```python
from build123d import *

# Parameters (mm, degrees)
EXTRUDE_1_DEPTH      = 1.4
EXTRUDE_1_DEPTH_BACK = 1.935048816
MM_1_D               = 1
MM_1_DEPTH           = 3.69956969
MM_1_TIP             = 0.30043031
MM_2_D               = 1
MM_2_DEPTH           = 3.69956969
MM_2_TIP             = 0.30043031
EXTRUDE_4_DEPTH      = 4
EXTRUDE_4_DEPTH_BACK = 7
CUT_EXTRUDE_4_DEPTH  = 4


with BuildPart() as part:
    # 草图1 → 凸台-拉伸1 (new body, two sides)
    with BuildSketch(Plane.XY) as extrude_1_sk:
        with BuildLine():
            Line((-14, 10.976009084), (64.784112274, 10.976009084))
            ThreePointArc((64.784112274, 10.976009084), (69.784112274, 5.976009084), (64.784112274, 0.976009084))
            Line((64.784112274, 0.976009084), (-14, 0.976009084))
            ThreePointArc((-14, 0.976009084), (-19, 5.976009084), (-14, 10.976009084))
        make_face()
        with BuildLine():
            Line((21.676320512, 3.476009084), (-1.323679488, 3.476009084))
            ThreePointArc((-1.323679488, 3.476009084), (-3.823679488, 5.976009084), (-1.323679488, 8.476009084))
            Line((-1.323679488, 8.476009084), (21.676320512, 8.476009084))
            ThreePointArc((21.676320512, 8.476009084), (24.176320512, 5.976009084), (21.676320512, 3.476009084))
        make_face(mode=Mode.SUBTRACT)
    extrude(amount=EXTRUDE_1_DEPTH)
    extrude(extrude_1_sk.sketch, amount=-EXTRUDE_1_DEPTH_BACK)

    # 大小mm 暗销孔1
    with Locations(Plane(origin=(0, 0, -1.935048816), x_dir=(-1, 0, 0), z_dir=(0, 0, -1))):
        with Locations((14, 5.976009084)):
            Hole(MM_1_D / 2, depth=MM_1_DEPTH)
            with Locations((0, 0, -(MM_1_DEPTH + MM_1_TIP / 2))):  # 118° drill point
                Cone(0, MM_1_D / 2, MM_1_TIP, mode=Mode.SUBTRACT)

    # 大小mm 暗销孔2
    with Locations(Plane(origin=(0, 0, -1.935048816), x_dir=(-1, 0, 0), z_dir=(0, 0, -1))):
        with Locations((-64.784112274, 5.976009084)):
            Hole(MM_2_D / 2, depth=MM_2_DEPTH)
            with Locations((0, 0, -(MM_2_DEPTH + MM_2_TIP / 2))):  # 118° drill point
                Cone(0, MM_2_D / 2, MM_2_TIP, mode=Mode.SUBTRACT)

    # 草图11 → 凸台-拉伸4 (add, two sides)
    with BuildSketch(Plane.XY.offset(1.4)) as extrude_4_sk:
        with BuildLine():
            Line((64.784112274, 10.976009084), (75.11027427, 10.181945777))
            Line((75.11027427, 10.181945777), (68.706480161, 6.265649051))
            Line((68.706480161, 6.265649051), (69.231074418, 4.88985116))
            Line((69.231074418, 4.88985116), (75.876804715, 9.001268784))
            Line((75.876804715, 9.001268784), (76.348764637, 8.189866665))
            Line((76.348764637, 8.189866665), (64.784112274, 0.976009084))
            ThreePointArc((64.784112274, 0.976009084), (65.998123298, 5.976009084), (64.784112274, 10.976009084))
        make_face()
    extrude(amount=EXTRUDE_4_DEPTH)
    extrude(extrude_4_sk.sketch, amount=-EXTRUDE_4_DEPTH_BACK)

    # 草图12 → 切除-拉伸4 (cut)
    with BuildSketch(Plane.XY.offset(1.4)):
        Polygon((69.702654004, 6.874867944), (68.706480161, 6.265649051), (69.231074418, 4.88985116), (69.722566431, 5.193915399), (71.19681176, 6.105965386), align=None)
        Polygon((64.784112274, 0.976009084), (69.274656978, 3.777143865), (71.000307029, 3.200660754), (64.195477274, -1.252602435), align=None)
    extrude(amount=-CUT_EXTRUDE_4_DEPTH, mode=Mode.SUBTRACT)


solid = part.part
```
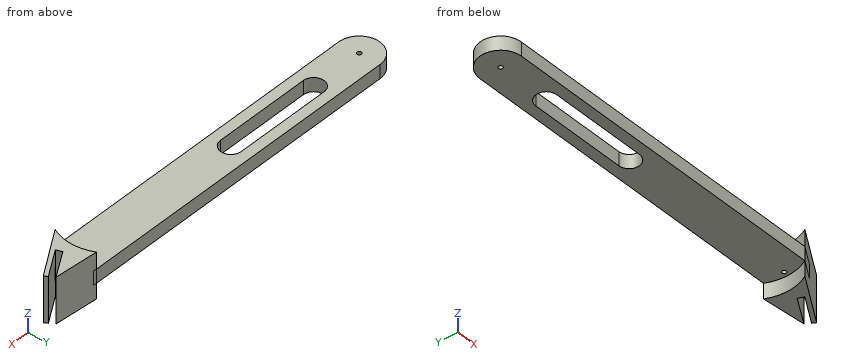
Verification items for the finished model (mm, model axes). Round coordinates to 2 decimals unless told otherwise and drop trailing zeros. Write each loop counter-clockwise with the first axis right and the second up, starting at its lowest first coordinate (ties: lowest second). Pieces come first, ordered by that corner, then holes.
1. Section check A-A on x = 9.5. Enter the section's corners in (y, z).
2. Gauge pin test, flat ends, axial feed: P1, Ø2, axis at x = 55, y = 4, coming from the -Z side; P2, Ø3, axis at y = 7.5, z = 3.5, coming from the +X side; P3, Ø3, axis at y = 2.5, z = 3, coming from the -X side; P4, Ø3, axis at y = 3.5, z = 0, coming from the -X side. Record the tip position at first contact, or that the pin passes through.
3. Scan lines: L1, parallel to Y at x = -14, z = 0.6; L2, parallel to Z at x = 17.5, y = 8.75; L3, parallel to X at y = 5.75, z = -4.25. Record each from-to range of solid material in increasing order.
4. Section check B-B on z = 2.75. Enter the section's corners in (x, y).
Answer:
1. outline: (0.98, -1.94) - (3.48, -1.94) - (3.48, 1.4) - (0.98, 1.4) - close; (8.48, -1.94) - (10.98, -1.94) - (10.98, 1.4) - (8.48, 1.4) - close
2. P1: stops at z = -1.94
2. P2: stops at x = 76.35
2. P3: stops at x = 64.8
2. P4: stops at x = -18.9
3. L1: y = 0.98 to 5.48, 6.48 to 10.98
3. L2: z = -1.94 to 1.4
3. L3: x = 66 to 68.9, 70.62 to 72.44
4. outline: (64.78, 0.98) - (76.35, 8.19) - (75.88, 9) - (69.23, 4.89) - (68.71, 6.27) - (75.11, 10.18) - (64.78, 10.98) arc R10.9 cw to start
